```python
from build123d import *

# Parameters (mm, degrees)
SKETCH1_R               = 2.25
BOSS_EXTRUDE1_DEPTH     = 10
BOSS_EXTRUDE3_DEPTH     = 70
BOSS_EXTRUDE3_2_DEPTH   = 70
SKETCH4_R               = 3.5
BOSS_EXTRUDE4_DEPTH     = 10
BOSS_EXTRUDE5_DEPTH     = 8.5
FILLET2_R               = 2
FILLET3_R               = 10
CUT_EXTRUDE1_DEPTH      = 10
CUT_EXTRUDE1_DEPTH_BACK = 125.104039016
SKETCH7_R               = 3.25


with BuildPart() as part:
    # Sketch1 → Boss-Extrude1 (new body)
    with BuildSketch(Plane.XY):
        with BuildLine():
            Line((15, 19.25), (-15, 19.25))
            Line((-15, 19.25), (-30, 19.25))
            Line((-30, 19.25), (-40, 19.25))
            ThreePointArc((-40, 19.25), (-43.535533906, 17.785533906), (-45, 14.25))
            Line((-45, 14.25), (-45, -14.25))
            ThreePointArc((-45, -14.25), (-43.535533906, -17.785533906), (-40, -19.25))
            Line((-40, -19.25), (-30, -19.25))
            Line((-30, -19.25), (-15, -19.25))
            Line((-15, -19.25), (-8.5, -19.25))
            Line((-8.5, -19.25), (-8.5, -16.75))
            Line((-8.5, -16.75), (-8.5, -11.437329234))
            ThreePointArc((-8.5, -11.437329234), (0, 14.25), (8.5, -11.437329234))
            Line((8.5, -11.437329234), (8.5, -16.75))
            Line((8.5, -16.75), (8.5, -19.25))
            Line((8.5, -19.25), (15, -19.25))
            Line((15, -19.25), (30, -19.25))
            Line((30, -19.25), (40, -19.25))
            ThreePointArc((40, -19.25), (43.535533906, -17.785533906), (45, -14.25))
            Line((45, -14.25), (45, 14.25))
            ThreePointArc((45, 14.25), (43.535533906, 17.785533906), (40, 19.25))
            Line((40, 19.25), (30, 19.25))
            Line((30, 19.25), (15, 19.25))
        make_face()
        with Locations((-15, -15)):
            Circle(SKETCH1_R, mode=Mode.SUBTRACT)
        with Locations((15, -15)):
            Circle(SKETCH1_R, mode=Mode.SUBTRACT)
        with Locations((-15, 15)):
            Circle(SKETCH1_R, mode=Mode.SUBTRACT)
        with Locations((15, 15)):
            Circle(SKETCH1_R, mode=Mode.SUBTRACT)
    extrude(amount=BOSS_EXTRUDE1_DEPTH)


with BuildPart() as body_2:
    # Sketch2 → Boss-Extrude3 (new body)
    with BuildSketch(Plane.XY.offset(10)):
        with BuildLine():
            Line((-45, 14.25), (-45, -14.25))
            ThreePointArc((-45, -14.25), (-43.535533906, -17.785533906), (-40, -19.25))
            Line((-40, -19.25), (-28, -19.25))
            Line((-28, -19.25), (-28, 0))
            Line((-28, 0), (-28, 19.25))
            Line((-28, 19.25), (-40, 19.25))
            ThreePointArc((-40, 19.25), (-43.535533906, 17.785533906), (-45, 14.25))
        make_face()
    extrude(amount=BOSS_EXTRUDE3_DEPTH)

    # Sketch4 → Boss-Extrude4 (add)
    with BuildSketch(Plane.XY.offset(80)):
        with BuildLine():
            Line((-45, 14.25), (-45, -14.25))
            ThreePointArc((-45, -14.25), (-43.535533906, -17.785533906), (-40, -19.25))
            Line((-40, -19.25), (-8.5, -19.25))
            Line((-8.5, -19.25), (-8.5, -11.437329234))
            ThreePointArc((-8.5, -11.437329234), (0, 14.25), (8.5, -11.437329234))
            Line((8.5, -11.437329234), (8.5, -19.25))
            Line((8.5, -19.25), (40, -19.25))
            ThreePointArc((40, -19.25), (43.535533906, -17.785533906), (45, -14.25))
            Line((45, -14.25), (45, 14.25))
            ThreePointArc((45, 14.25), (43.535533906, 17.785533906), (40, 19.25))
            Line((40, 19.25), (-40, 19.25))
            ThreePointArc((-40, 19.25), (-43.535533906, 17.785533906), (-45, 14.25))
        make_face()
        with Locations((-21.5, 0)):
            Circle(SKETCH4_R, mode=Mode.SUBTRACT)
    extrude(amount=BOSS_EXTRUDE4_DEPTH)

    # Sketch6 → Boss-Extrude5 (add)
    with BuildSketch(Plane.XY.offset(90)):
        with BuildLine():
            Line((-40, -19.25), (-8.5, -19.25))
            Line((-8.5, -19.25), (-8.5, -11.437329234))
            ThreePointArc((-8.5, -11.437329234), (0, 14.25), (8.5, -11.437329234))
            Line((8.5, -11.437329234), (8.5, -19.25))
            Line((8.5, -19.25), (40, -19.25))
            ThreePointArc((40, -19.25), (43.535533906, -17.785533906), (45, -14.25))
            Line((45, -14.25), (45, 14.25))
            ThreePointArc((45, 14.25), (43.535533906, 17.785533906), (40, 19.25))
            Line((40, 19.25), (-40, 19.25))
            ThreePointArc((-40, 19.25), (-43.535533906, 17.785533906), (-45, 14.25))
            Line((-45, 14.25), (-45, -14.25))
            ThreePointArc((-45, -14.25), (-43.535533906, -17.785533906), (-40, -19.25))
        make_face()
        Polygon((-16.7, 0), (-19.1, 4.156921938), (-23.9, 4.156921938), (-26.3, 0), (-23.9, -4.156921938), (-19.1, -4.156921938), align=None, mode=Mode.SUBTRACT)
    extrude(amount=BOSS_EXTRUDE5_DEPTH)


with BuildPart() as body_3:
    # Sketch2 → Boss-Extrude3 2 (new body)
    with BuildSketch(Plane.XY.offset(10)):
        with BuildLine():
            Line((40, -19.25), (28, -19.25))
            Line((28, -19.25), (28, 0))
            Line((28, 0), (28, 19.25))
            Line((28, 19.25), (40, 19.25))
            ThreePointArc((40, 19.25), (43.535533906, 17.785533906), (45, 14.25))
            Line((45, 14.25), (45, -14.25))
            ThreePointArc((45, -14.25), (43.535533906, -17.785533906), (40, -19.25))
        make_face()
    extrude(amount=BOSS_EXTRUDE3_2_DEPTH)


with BuildPart() as part_1:
    add(part.part)

    # Combine1: union body 2, body 3
    add(body_2.part)
    add(body_3.part)

    # Fillet2
    fillet2_edges = [part_1.edges().sort_by_distance(p)[0] for p in [
        (-28, 0, 80),
    ]]
    fillet(fillet2_edges, radius=FILLET2_R)

    # Fillet3
    fillet3_edges = [part_1.edges().sort_by_distance(p)[0] for p in [
        (28, 0, 80),
        (-28, 0, 10),
        (28, 0, 10),
    ]]
    fillet(fillet3_edges, radius=FILLET3_R)

    # Sketch7 → Cut-Extrude1 (cut, two sides: drawn at the far end of the back side and taken through both)
    with BuildSketch(Plane(origin=(-28, 0, 0), x_dir=(0, 0, -1), z_dir=(1, 0, 0)).offset(-CUT_EXTRUDE1_DEPTH_BACK)):
        with Locations(Location((-20, -11.25, 0), (0, 0, 247.380135052))):
            Circle(SKETCH7_R)
    extrude(amount=CUT_EXTRUDE1_DEPTH + CUT_EXTRUDE1_DEPTH_BACK, mode=Mode.SUBTRACT)


solid = part_1.part
```
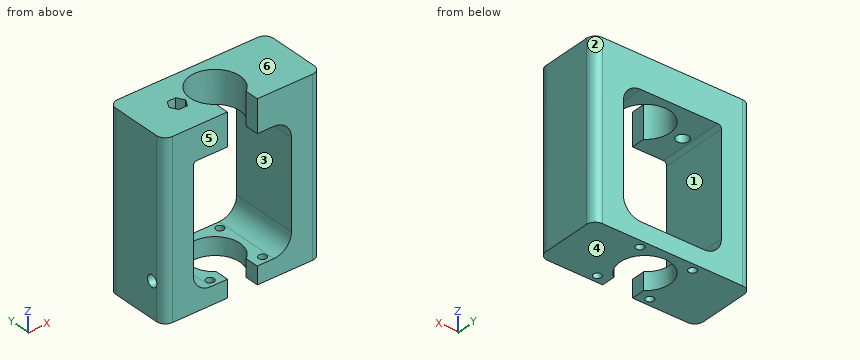
Input: part model. Units: mm. Frame: model coordinates. Face numbers are marked on the shaded views. A direction names the side the tool comes from. Coordinates: 2 decimals unless noted, no trailing zeros. Write each loop counter-clockwise with the first axis right and the second up, starting at its lowest first coordinate (ties: lowest second). Pieces come first, ordered by that corner, then holes. Notation, with made-up numbers: (81, -12) - (89, -12) arc R16 cw to (89, -6) - close; hole circle Ø10 at (24, -14). An arc over 180 degrees is marked (long way). Put each result on its own line as item: value. Start each with the question number.
1) Mould query, pull axis Z, two halves, no side actions, for the marked faces 3, 4, 5 and 6. Classes: pulls with the +Z half, pulls with the -Z half, needs draft (parallel to the pull), parting line crosses it, or undercut.
2) Reachability of the marked faces 1 and 2 from +Z, -Z, +X, -X, +Y, -Y: full face, straight path, thin tool, end or side. Return the list, or none.
3) Cut plane C-C (y = -5.5). Return the cut outline in (x, z), plus the area to 3 significant figures.
4) Cut plane B-B (z = 12.5). Return the cut outline in (x, y).
5) Cut plane D-D (x = -21.5). Return the cut outline in (y, z), plus the area to 3 significant figures.
6) Ray query, L1, parallel to Y at x = 15, z = 7; L2, parallel to X at y = -1, z = 70; L3, parallel to Z at x = -17.5, y = 17. Return the intervals inside material, ascending.
7) Cut plane A-A (x = 0). Return the cut outline in (y, z).
8) Contact query for flat-ended pins moving along their axis: pin 1 (5.5 mm diameter, centred on x = -21.5, y = 0, fed in from +Z); pin 2 (4 mm diameter, centred on y = -17.5, z = 85.5, fed in from -X); pin 3 (18 mm diameter, centred on x = 2.5, y = -2.5, fed in from +Z). Output: stop coordinate, or through.
Resolved:
1. face 3: undercut
1. face 4: pulls with the -Z half
1. face 5: needs draft
1. face 6: pulls with the +Z half
2. face 1: +Y, -Y
2. face 2: +Z, -Z, +X, +Y
3. outline: (-45, 0) - (-13.15, 0) - (-13.15, 10) - (-18, 10) arc R10 cw to (-28, 20) - (-28, 78) arc R2 cw to (-26, 80) - (-13.15, 80) - (-13.15, 98.5) - (-45, 98.5) - close; (13.15, 0) - (45, 0) - (45, 98.5) - (13.15, 98.5) - (13.15, 80) - (18, 80) arc R10 cw to (28, 70) - (28, 20) arc R10 cw to (18, 10) - (13.15, 10) - close
3. area: 4,260 mm2
4. outline: (-45, -14.25) arc R5 ccw to (-40, -19.25) - (-24.61, -19.25) - (-24.61, 19.25) - (-40, 19.25) arc R5 ccw to (-45, 14.25) - close; (24.61, -19.25) - (40, -19.25) arc R5 ccw to (45, -14.25) - (45, 14.25) arc R5 ccw to (40, 19.25) - (24.61, 19.25) - close
5. outline: (-19.25, 0) - (19.25, 0) - (19.25, 10.63) - (-19.25, 10.63) - close; (-19.25, 80) - (-3.5, 80) - (-3.5, 90) - (-4.16, 90) - (-4.16, 98.5) - (-19.25, 98.5) - close; (3.5, 80) - (19.25, 80) - (19.25, 98.5) - (4.16, 98.5) - (4.16, 90) - (3.5, 90) - close
5. area: 981 mm2
6. L1: y = -19.25 to -17.25, -12.75 to 12.75, 17.25 to 19.25
6. L2: x = -45 to -28, 28 to 45
6. L3: z = 0 to 10, 80 to 98.5
7. outline: (14.25, 0) - (19.25, 0) - (19.25, 10) - (14.25, 10) - close; (14.25, 80) - (19.25, 80) - (19.25, 98.5) - (14.25, 98.5) - close
8. pin 1: stops at z = 12.19
8. pin 2: stops at x = -44.84
8. pin 3: passes through
